The model under review builds one solid part; all positions refer to its coordinate system, in mm. A direction names the side the tool comes from. Give positions to 0.01 mm unless a question says otherwise; leave off trailing zeros. Loops run counter-clockwise (first coordinate to the right, second up) from the corner with the lowest first, then second, coordinate; pieces in that order, holes last. Notation, with made-up numbers: M 79.25,-10.75 L 108.25,-10.75 A16 cw 108.25,-3.75 Z; hole C -35.75,35 d11. An arc over 180 degrees is marked long. Return JSON: item names as keys, results as strings. Group by question number.
```python
from build123d import *

# Parameters (mm, degrees)
CROQUIS2_W              = 168
CROQUIS2_H              = 66.31
SALIENTE_EXTRUIR1_DEPTH = 5
CROQUIS3_W              = 2.5
CROQUIS3_H              = 10.2
SALIENTE_EXTRUIR3_DEPTH = 5
CROQUIS5_W              = 10.2
CROQUIS5_H              = 5.2
CORTAR_EXTRUIR2_DEPTH   = 181.68208572
CROQUIS7_W              = 8
CROQUIS7_H              = 2.5
CORTAR_EXTRUIR3_DEPTH   = 181.68208572
SKETCH1_W               = 2.5
SKETCH1_H               = 10.2
BOSS_EXTRUDE1_DEPTH     = 5


with BuildPart() as part:
    # Croquis2 → Saliente-Extruir1 (new body)
    with BuildSketch(Plane.XY):
        with Locations((84, 33.155)):
            Rectangle(CROQUIS2_W, CROQUIS2_H)
    extrude(amount=-SALIENTE_EXTRUIR1_DEPTH)

    # Croquis3 → Saliente-Extruir3 (add)
    with BuildSketch(Plane.XY):
        with Locations((2.5, 31.31)):
            Rectangle(CROQUIS3_W, CROQUIS3_H)
    extrude(amount=SALIENTE_EXTRUIR3_DEPTH)

    # Croquis5 → Cortar-Extruir2 (cut, through all)
    with BuildSketch(Plane.XY):
        with Locations((103, 42.6)):
            Rectangle(CROQUIS5_W, CROQUIS5_H)
        with Locations((53, 42.6)):
            Rectangle(CROQUIS5_W, CROQUIS5_H)
    extrude(amount=-CORTAR_EXTRUIR2_DEPTH, mode=Mode.SUBTRACT)

    # Croquis7 → Cortar-Extruir3 (cut, through all)
    with BuildSketch(Plane.XY):
        with Locations((30, 2.5)):
            Rectangle(CROQUIS7_W, CROQUIS7_H)
        with Locations((138, 2.5)):
            Rectangle(CROQUIS7_W, CROQUIS7_H)
    extrude(amount=-CORTAR_EXTRUIR3_DEPTH, mode=Mode.SUBTRACT)

    # Sketch1 → Boss-Extrude1 (add)
    with BuildSketch(Plane.XY):
        with Locations((165.5, 31.31)):
            Rectangle(SKETCH1_W, SKETCH1_H)
    extrude(amount=BOSS_EXTRUDE1_DEPTH)


solid = part.part
```
(1) For probe 1 along Y at (x, z) = (108, -1); probe 2 along X at (y, z) = (32, 0.5); probe 3 along Z at (x, y) = (54.5, 51.5), list the stretches that pass through material, from the lowest coordinate up.
(2) Mouldability with a two-part tool opening along X and no side actions: class faces 1 (the flat face through (83, 0, -2)), 2 (the flat face through (30, 3.75, -2)), 3 (the flat face through (0, 33, -2)), 4 (the flat face through (164.25, 31, 2)) as released by +X, released by -X, zero draft, split by the parting line, or undercut.
(3) Add section B-B (x = 138). Write out the cut boundary in (y, z).
(4) Add section A-A (y = 42.5). Write out the cut boundary in (x, z), and give its area (3 significant figures).
(5) Add section C-C (z = 2). Write out the cut boundary in (x, y).
(6) For pin 1 (2 mm diameter, centred on y = 2, z = -1.5, fed in from -X); pin 2 (1 mm diameter, centred on y = 53.5, z = 1.5, fed in from -X); pin 3 (0.8 mm diameter, centred on x = 165.5, z = 2, fed in from +Y); pin 4 (1.5 mm diameter, centred on y = 29.5, z = 2.5, fed in from +X), all flat-tipped, find the tip position at first contact; note any pin that passes through.
(7) For faces 5 (the flat face through (30, 1.25, -2)), 6 (the flat face through (83, 34, -5)), 7 (the flat face through (166.75, 31, 2)), 8 (the flat face through (1.25, 31, 2)), 9 (the flat face through (168, 33, -2)), list the 3-axis set-ups (+Z, -Z, +X, -X, +Y, -Y) from which the entire face can be reached by the end or side of a thin tool; tool diameter is ignored.
(8) Add section D-D (y = 34). Write out the cut boundary in (x, z), and give its area (3 significant figures).
Verdict:
{
 "1": {"probe 1": "y = 0 to 40, 45.2 to 66.31", "probe 2": "x = 1.25 to 3.75, 164.25 to 166.75", "probe 3": "z = -5 to 0"},
 "2": {"face 1": "zero draft", "face 2": "undercut", "face 3": "released by -X", "face 4": "undercut"},
 "3": {"outline": "M 0,-5 L 1.25,-5 L 1.25,0 L 0,0 Z; M 3.75,-5 L 66.31,-5 L 66.31,0 L 3.75,0 Z"},
 "4": {"outline": "M 0,-5 L 47.9,-5 L 47.9,0 L 0,0 Z; M 58.1,-5 L 97.9,-5 L 97.9,0 L 58.1,0 Z; M 108.1,-5 L 168,-5 L 168,0 L 108.1,0 Z", "area": "738 mm²"},
 "5": {"outline": "M 1.25,26.21 L 3.75,26.21 L 3.75,36.41 L 1.25,36.41 Z; M 164.25,26.21 L 166.75,26.21 L 166.75,36.41 L 164.25,36.41 Z"},
 "6": {"pin 1": "stops at x = 0", "pin 2": "passes through", "pin 3": "stops at y = 36.41", "pin 4": "stops at x = 166.75"},
 "7": {"face 5": "+Z, -Z", "face 6": "-Z, +X, -X, +Y, -Y", "face 7": "+Z, +X, +Y, -Y", "face 8": "+Z, -X, +Y, -Y", "face 9": "+Z, -Z, +X, +Y, -Y"},
 "8": {"outline": "M 0,-5 L 168,-5 L 168,0 L 166.75,0 L 166.75,5 L 164.25,5 L 164.25,0 L 3.75,0 L 3.75,5 L 1.25,5 L 1.25,0 L 0,0 Z", "area": "865 mm²"}
}
